from build123d import *
from OCP.BRepFilletAPI import BRepFilletAPI_MakeChamfer

# Parameters (mm, degrees)
SKETCH_1_W                   = 40
SKETCH_1_H                   = 15
EXTRUDE_1_DEPTH              = 60
SKETCH_3_W                   = 40
SKETCH_3_H                   = 40
EXTRUDE_2_DEPTH              = 10
HOLE_WIZARD_M4_1_D           = 4.5
HOLE_WIZARD_M4_1_CBORE_D     = 8
HOLE_WIZARD_M4_1_CBORE_DEPTH = 4.4
CHAMFER_1_SIZE               = 5
CHAMFER_2_SIZE               = 2
CUT_EXTRUDE_2_DEPTH          = 50
CHAMFER_3_SIZE               = 1
CHAMFER_3_SIZE2              = 0.84312817
CUT_EXTRUDE_3_DEPTH          = 10
CHAMFER_4_SIZE               = 1


with BuildPart() as part:
    # 草图1 → 凸台-拉伸1 (new body)
    with BuildSketch(Plane(origin=(0, 0, 0), x_dir=(1, 0, 0), z_dir=(0, 1, 0))):
        Rectangle(SKETCH_1_W, SKETCH_1_H)
    extrude(amount=EXTRUDE_1_DEPTH)

    # 草图3 → 凸台-拉伸2 (add)
    with BuildSketch(Plane(origin=(0, 60, 0), x_dir=(1, 0, 0), z_dir=(0, 1, 0))):
        with Locations((0, -12.5)):
            Rectangle(SKETCH_3_W, SKETCH_3_H)
    extrude(amount=EXTRUDE_2_DEPTH)

    # M4 六角凹头螺钉的柱形沉头孔1 (through all)
    with Locations(Plane(origin=(0, 60, 0), x_dir=(-1, 0, 0), z_dir=(0, -1, 0))):
        with Locations((12, -11.5), (-12, -11.5), (12, -27.5), (-12, -27.5)):
            CounterBoreHole(HOLE_WIZARD_M4_1_D / 2, HOLE_WIZARD_M4_1_CBORE_D / 2, HOLE_WIZARD_M4_1_CBORE_DEPTH)

    # 倒角1
    chamfer_1_edges = [part.edges().sort_by_distance(p)[0] for p in [
        (0, 70, -7.5),
    ]]
    chamfer(chamfer_1_edges, length=CHAMFER_1_SIZE)

    # 倒角2
    chamfer_2_edges = [part.edges().sort_by_distance(p)[0] for p in [
        (-20, 32.5, -7.5),
        (20, 32.5, -7.5),
    ]]
    chamfer(chamfer_2_edges, length=CHAMFER_2_SIZE)

    # 草图7 → 切除-拉伸2 (cut)
    with BuildSketch(Plane.XZ):
        Polygon((-6, -3.5), (4, -3.5), (25.464703606, 1.062463596), (25.464703606, 11.878030996), (-23.00207338, 11.878030996), (-23.00207338, 0.113902259), align=None)
    extrude(amount=-CUT_EXTRUDE_2_DEPTH, mode=Mode.SUBTRACT)

    # 倒角3: one chamfer whose edges measure the first distance from different faces: ONE call of the kernel's chamfer builder (chamfer() names one face for all edges)
    chamfer_3_edges_1 = [part.edges().sort_by_distance(p)[0] for p in [
        (-20, 25, -0.524208137),
    ]]
    chamfer_3_side_1 = [part.faces().sort_by_distance(p)[0] for p in [
        (-13, 25, -2.012104068),
    ]]
    chamfer_3_edges_2 = [part.edges().sort_by_distance(p)[0] for p in [
        (20, 25, -0.099095013),
    ]]
    chamfer_3_side_2 = [part.faces().sort_by_distance(p)[0] for p in [
        (12, 25, -1.799547507),
    ]]
    chamfer_3 = BRepFilletAPI_MakeChamfer(part.part.solid().wrapped)
    for e in chamfer_3_edges_1:
        chamfer_3.Add(CHAMFER_3_SIZE, CHAMFER_3_SIZE2, e.wrapped, chamfer_3_side_1[0].wrapped)  # the first distance lies on this face
    for e in chamfer_3_edges_2:
        chamfer_3.Add(CHAMFER_3_SIZE, CHAMFER_3_SIZE2, e.wrapped, chamfer_3_side_2[0].wrapped)  # the first distance lies on this face
    add(Compound.cast(chamfer_3.Shape()), mode=Mode.REPLACE)

    # 草图8 → 切除-拉伸3 (cut)
    with BuildSketch(Plane.XZ.offset(-50)):
        Polygon((-10, 7.5), (-5, 2.5), (5, 2.5), (10, 7.5), align=None)
    extrude(amount=-CUT_EXTRUDE_3_DEPTH, mode=Mode.SUBTRACT)

    # 倒角4
    chamfer_4_edges = [part.edges().sort_by_distance(p)[0] for p in [
        (-20, 65, 32.5),
        (20, 65, 32.5),
        (-20, 55, 7.5),
        (20, 55, 7.5),
    ]]
    chamfer(chamfer_4_edges, length=CHAMFER_4_SIZE)


solid = part.part
The listing builds one solid part. Answer for the finished solid, in the listing's coordinates (mm). A direction names the side the tool comes from. Coordinates: 2 decimals unless noted, no trailing zeros. Loops run counter-clockwise (first coordinate to the right, second up) from the corner with the lowest first, then second, coordinate; pieces in that order, holes last.
1) Flat-ended cylindrical pins translate along their axes: pin 1 Ø6.5 at (x, z) = (10, 11) entering from -Y; pin 2 Ø5.5 at (x, z) = (3, -0.5) entering from -Y; pin 3 Ø12 at (x, y) = (-7, 29.5) entering from +Z. Find the tip coordinate at first contact, or state that the pin passes through.
2) Find section D-D on y = 22. Write down the section's boundary in (x, z), then the cut area to 3 significant figures.
3) A tool of negligible diameter and unlimited length cuts with its end or side. For faces 4 (the face through (0, 60, 17)), 5 (the face through (-14, 64.4, 13)), 6 (the face through (-15, 55, 7.5)), from which of +Z, -Z, +X, -X, +Y, -Y can it reach the whole face along a straight path? Write none if from no direction.
4) Find the intervals of material crossed by L1, parallel to X at y = 68.65, z = 27.5; L2, parallel to X at y = 61.9, z = 27.5; L3, parallel to Z at x = 12, y = 68.7, in increasing order.
5) Determine the mould class of faces 1 (the face through (20, 53, 6)), 2 (the face through (0, 50, 2)), 3 (the face through (14, 55, 7.5)) for opening direction X: pulls with the +X half, pulls with the -X half, needs draft (parallel to the pull), parting line crosses it, or undercut.
6) Find section C-C on x = 3. Write down the section's boundary in (y, z), then the cut area to 4 significant figures.
7) Find section A-A on z = 27.5. Write down the section's boundary in (x, y), then the cut area to 3 significant figures.
8) Find section B-B on y = 63. Write down the section's boundary in (x, z).
Values:
1. pin 1: stops at y = 60
1. pin 2: stops at y = 50
1. pin 3: stops at z = -2.01
2. outline: (-20, -5.5) - (-18, -7.5) - (18, -7.5) - (20, -5.5) - (20, -0.94) - (19.02, -0.31) - (4, -3.5) - (-6, -3.5) - (-19.02, -0.73) - (-20, -1.37) - close
2. area: 203 mm2
3. face 4: +Z, -Y
3. face 5: -Y
3. face 6: +Z, +X, -X, -Y
4. L1: x = -20 to -14.25, -9.75 to 9.75, 14.25 to 20
4. L2: x = -20 to -16, -8 to 8, 16 to 20
4. L3: z = -3.8 to 9.25, 13.75 to 25.25, 29.75 to 32.5
5. face 1: pulls with the +X half
5. face 2: undercut
5. face 3: needs draft
6. outline: (0, -7.5) - (65, -7.5) - (70, -2.5) - (70, 32.5) - (60, 32.5) - (60, 2.5) - (50, 2.5) - (50, -3.5) - (0, -3.5) - close
6. area: 687.5 mm2
7. outline: (-20, 60) - (-16, 60) - (-16, 64.4) - (-14.25, 64.4) - (-14.25, 70) - (-20, 70) - close; (-9.75, 64.4) - (-8, 64.4) - (-8, 60) - (8, 60) - (8, 64.4) - (9.75, 64.4) - (9.75, 70) - (-9.75, 70) - close; (14.25, 64.4) - (16, 64.4) - (16, 60) - (20, 60) - (20, 70) - (14.25, 70) - close
7. area: 279 mm2
8. outline: (-20, -5.5) - (-18, -7.5) - (18, -7.5) - (20, -5.5) - (20, 31.5) - (19, 32.5) - (-19, 32.5) - (-20, 31.5) - close; hole circle Ø8 at (-12, 11.5); hole circle Ø8 at (-12, 27.5); hole circle Ø8 at (12, 11.5); hole circle Ø8 at (12, 27.5)
